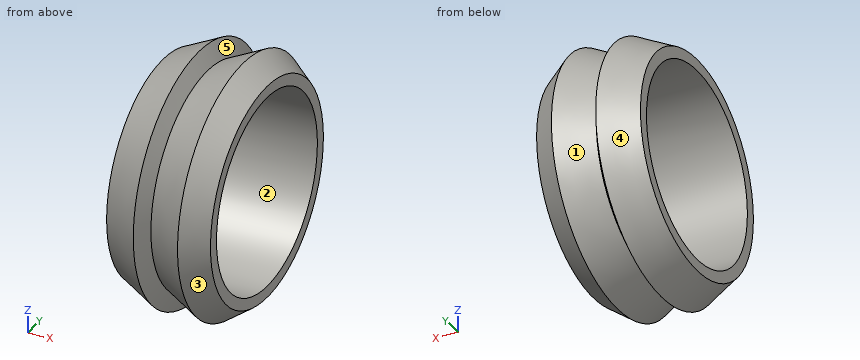
```python
from build123d import *

# Parameters (mm, degrees)
F2_R     = 6.532772
F3_DEPTH = 25.4


with BuildPart() as f1:
    # F0 (on Front) → F1 (revolve)
    with BuildSketch(Plane.XZ):
        Polygon((0, 7.308824), (0, 0), (6.985, 0), (6.985, 7.308824), (2.977107, 7.308824), align=None)
        Polygon((2.40231, 8.483916), (0, 7.308824), (2.977107, 7.308824), align=None)
        Polygon((2.977107, 7.308824), (6.985, 7.308824), (5.379418, 8.483916), align=None)
    revolve(axis=Axis((-6.382353, 0, 0), (-1, 0, 0)))

    # F2 (on face) → F3 (cut)
    with BuildSketch(Plane(origin=(0, 0, 0), x_dir=(0, -1, 0), z_dir=(-1, 0, 0))):
        Circle(F2_R)
    extrude(amount=-F3_DEPTH, mode=Mode.SUBTRACT)


solid = f1.part
```
Model file for the job. Use its own axes, mm. Face numbers are marked on the shaded views. A direction names the side the tool comes from. Coordinates: 2 decimals unless noted, no trailing zeros. Loops run counter-clockwise (first coordinate to the right, second up) from the corner with the lowest first, then second, coordinate; pieces in that order, holes last. Notation, with made-up numbers: (16.25, 83.5) - (36.25, 83.5) arc R15 ccw to (36.25, 110.5) - close; hole circle Ø2 at (-10, -27.75). An arc over 180 degrees is marked (long way). Answer as a JSON object with one key per item and string values. Group by question number.
(1) Cut at D-D (x = 4). Give the cut face in (y, z), then the cut area to 3 significant figures.
(2) Cut at C-C (x = 1). Give the cut face in (y, z).
(3) Two-plate mould, pull along X, no slides. Class the marked faces 3, 4 and 5: released by +X, released by -X, zero draft, split by the parting line, or undercut.
(4) Flat gauge pins, fed straight in: pin 1 (3 mm diameter, centred on x = 5, z = 2, fed in from -Y); pin 2 (2 mm diameter, centred on x = 4, z = 3, fed in from +Y). Where does each tip first touch, or does it go through?
(5) Probe line 1 along Y through (x, z) = (2.25, 1.5); line 2 along Y through (x, z) = (4.5, 1.25); line 3 along Z through (x, y) = (3.75, 0). List the from-to ranges inside material, lowest first.
(6) Tool access for the marked faces 1 and 2: list every direction of +Z, -Z, +X, -X, +Y, -Y with a clear straight run to the whole face (end or side of a thin tool).
(7) Cut at A-A (y = 0). Give the cut face in (x, z) (3 decimals).
Geometry says:
{
 "1": {"outline": "circle Ø15.62 at (0, 0); hole circle Ø13.07 at (0, 0)", "area": "57.5 mm^2"},
 "2": {"outline": "circle Ø15.6 at (0, 0); hole circle Ø13.07 at (0, 0)"},
 "3": {"face 3": "released by +X", "face 4": "released by -X", "face 5": "undercut"},
 "4": {"pin 1": "stops at y = -8.47", "pin 2": "stops at y = 7.84"},
 "5": {"line 1": "y = -8.27 to -6.36, 6.36 to 8.27", "line 2": "y = -7.96 to -6.41, 6.41 to 7.96", "line 3": "z = -7.69 to -6.53, 6.53 to 7.69"},
 "6": {"face 1": "none", "face 2": "+X, -X"},
 "7": {"outline": "(0, -7.309) - (2.402, -8.484) - (2.977, -7.309) - (5.379, -8.484) - (6.985, -7.309) - (6.985, -6.533) - (0, -6.533) - close; (0, 6.533) - (6.985, 6.533) - (6.985, 7.309) - (5.379, 8.484) - (2.977, 7.309) - (2.402, 8.484) - (0, 7.309) - close"}
}
